from build123d import *

# Parameters (mm, degrees)
SKETCH1_R           = 1.262505146
BOSS_EXTRUDE1_DEPTH = 2.4


with BuildPart() as part:
    # Sketch1 → Boss-Extrude1 (new body)
    with BuildSketch(Plane.XY):
        Polygon((17, 25.571584313), (15, 25.571584313), (15, 27.971584313), (5, 27.971584313), (5, 25.571584313), (2, 25.571584313), (2, 22.204806168), (3.4, 22.204806168), (3.4, 19.704806168), (2, 19.704806168), (2, 15.571584313), (-2, 15.571584313), (-2, 19.704806168), (-3.4, 19.704806168), (-3.4, 22.204806168), (-2, 22.204806168), (-2, 25.571584313), (-5, 25.571584313), (-5, 27.971584313), (-15, 27.971584313), (-15, 25.571584313), (-17, 25.571584313), (-17, -24.428415687), (-1.5, -24.428415687), (-1.5, -17.028415687), (-6.1, -17.028415687), (-6.1, 5.571584313), (0, 5.571584313), (6.1, 5.571584313), (6.1, -17.028415687), (1.5, -17.028415687), (1.5, -24.428415687), (17, -24.428415687), align=None)
        with Locations((0, 8.071584313)):
            Circle(SKETCH1_R, mode=Mode.SUBTRACT)
    extrude(amount=BOSS_EXTRUDE1_DEPTH)


solid = part.part
Geometry: final body of the model. Coordinates: model frame, mm. A direction names the side the tool comes from. Round coordinates to 2 decimals unless told otherwise and drop trailing zeros. Loops run counter-clockwise (first coordinate to the right, second up) from the corner with the lowest first, then second, coordinate; pieces in that order, holes last. Notation, with made-up numbers: M 29,88 L 46,88 A14 ccw 46,104 Z; hole C 23.5,6.5 d6. An arc over 180 degrees is marked long. Put each result on its own line as item: value. Start each with the question number.
(1) Material intervals for line 1 along Y through (x, z) = (3, 0.35); line 2 along X through (y, z) = (20.5, 0.8); line 3 along Y through (x, z) = (0, 1.05), sorted ascending. Write a range as [from, to].
(2) Section query A-A (x = 0). Return loops of the section in (y, z), then the cut area to 3 significant figures.
(3) Set-up query: faces 5 (the face through (-2, 18, 1)), 6 (the face through (-10, 27.972, 1)), 7 (the face through (-9, -24.428, 1)), 8 (the face through (1.5, -21, 1)), 9 (the face through (-6.1, -6, 1)). Return all of +Z, -Z, +X, -X, +Y, -Y with unobstructed straight access to the full face (end or side cutting, diameter ignored); none if empty.
(4) Draft query along X for faces 1 (the face through (17, 0, 1)), 2 (the face through (16, 25.572, 1)), 3 (the face through (3.4, 21, 1)), 4 (the face through (5, 27, 1)). Return one class per face: +X half, -X half, draft (parallel to the pull), parting line (faces both ways), or undercut.
(5) Contact query for flat-ended pins moving along their axis: pin 1 Ø1.1 at (x, z) = (-2.5, 1.5) entering from +Y; pin 2 Ø1.2 at (y, z) = (27.5, 1.5) entering from +X. Output: stop coordinate, or through.
(6) Section query B-B (y = 1.5). Return loops of the section in (x, z).
Findings below:
1. line 1: y = [-24.43, -17.03], [5.57, 19.7], [22.2, 25.57]
1. line 2: x = [-17, -3.4], [3.4, 17]
1. line 3: y = [5.57, 6.81], [9.33, 15.57]
2. outline: M 5.57,0 L 6.81,0 L 6.81,2.4 L 5.57,2.4 Z; M 9.33,0 L 15.57,0 L 15.57,2.4 L 9.33,2.4 Z
2. area: 17.9 mm2
3. face 5: +Z, -Z, +Y
3. face 6: +Z, -Z, +X, -X, +Y
3. face 7: +Z, -Z, +X, -X, -Y
3. face 8: +Z, -Z, -Y
3. face 9: +Z, -Z
4. face 1: +X half
4. face 2: draft
4. face 3: undercut
4. face 4: undercut
5. pin 1: stops at y = 25.57
5. pin 2: stops at x = 15
6. outline: M -17,0 L -6.1,0 L -6.1,2.4 L -17,2.4 Z; M 6.1,0 L 17,0 L 17,2.4 L 6.1,2.4 Z
